The listing builds one solid part. Answer for the finished solid, in the listing's coordinates (mm). Face numbers are marked on the shaded views. Give positions to 0.01 mm unless a question says otherwise; leave off trailing zeros. Order: outer loops, then holes, each group sorted by start corner. A loop starts at its lowest first (then second) coordinate and runs counter-clockwise, first axis right, second up. Notation, with made-up numbers: (7.25, 17.5) - (16.25, 17.5) arc R27 ccw to (16.25, 33.5) - close; hole circle Ø8 at (7.25, 85). An arc over 180 degrees is marked (long way). Answer as a JSON object with one key per item and string values. Group by question number.
Q1. Consider line 1 (Y direction, x = 0, z = 2.7); line 2 (Z direction, x = 11, y = 2.25); line 3 (Z direction, x = 0, y = 2.5). Determine where each line is inside the solid, lowest interval first.
Q2. A cutting plane is placed at B-B, the plane z = 4. Give the vertices of the cut face in (x, y).
Q3. The mould has two halves that part along Y. Classify the marked faces 1, 2 and 3: released by +Y, released by -Y, zero draft, split by the parting line, or undercut.
Q4. A cutting plane is placed at A-A, the plane x = 13.5. Give the vertices of the cut face in (y, z).
Q5. Given pin 1 (0.8 mm diameter, centred on y = 3.5, z = 8, fed in from +X); pin 2 (3 mm diameter, centred on x = -14, y = 0, fed in from -Z); pin 3 (5 mm diameter, centred on x = -13, y = 2, fed in from +Z); pin 4 (5 mm diameter, centred on y = 3, z = 6.5, fed in from +X), each flat-ended and moving along its own axis, determine where each tip first touches the part or whether it passes through.
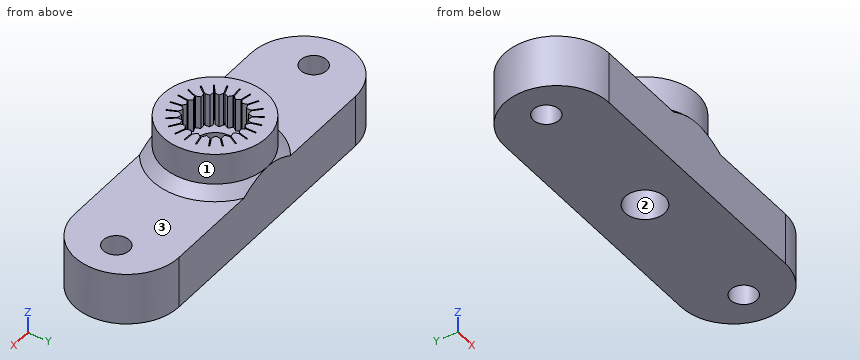
from build123d import *

# Parameters (mm, degrees)
EXTRUDE_1_DEPTH          = 5
SKETCH_6_R               = 5
EXTRUDE_3_DEPTH          = 4
CUT_EXTRUDE_5_DEPTH      = 3.2
CHAMFER_1_SIZE           = 1
CUT_EXTRUDE_6_DEPTH      = 21.303940504
CUT_EXTRUDE_6_DEPTH_BACK = 21.303940504
SKETCH_7_R               = 1.25
SKETCH_7_R_2             = 1.9


with BuildPart() as part:
    # ｽｹｯﾁ1 → ﾎﾞｽ - 押し出し1 (new body)
    with BuildSketch(Plane.XY):
        with BuildLine():
            Line((12.5, -5), (-12.5, -5))
            ThreePointArc((-12.5, -5), (-17.5, 0), (-12.5, 5))
            Line((-12.5, 5), (12.5, 5))
            ThreePointArc((12.5, 5), (17.5, 0), (12.5, -5))
        make_face()
    extrude(amount=EXTRUDE_1_DEPTH)

    # ｽｹｯﾁ6 → ﾎﾞｽ - 押し出し3 (add)
    with BuildSketch(Plane.XY.offset(5)):
        with Locations(Location((0, 0, 0), (0, 0, 270))):
            Circle(SKETCH_6_R)
    extrude(amount=EXTRUDE_3_DEPTH)

    # ｽｹｯﾁ5 → ｶｯﾄ - 押し出し5 (cut)
    with BuildSketch(Plane.XY.offset(9)):
        Polygon((-0.05, 2.95), (-0.05, 3.95), (0.05, 3.95), (0.05, 2.95), (0.362514094, 2.637485906), (0.747754611, 2.854095836), (1.017551382, 3.817013124), (1.11384311, 3.790033446), (0.844046339, 2.827116159), (1.060656269, 2.441875642), (1.490051682, 2.546516441), (2.009635632, 3.400935845), (2.095077573, 3.34897745), (1.575493623, 2.494558046), (1.680134421, 2.065162633), (2.121838437, 2.050073571), (2.852674402, 2.732626714), (2.920929716, 2.659543117), (2.190093752, 1.976989974), (2.17500469, 1.535285958), (2.596258142, 1.401586122), (3.484143361, 1.86165116), (3.530149865, 1.772862638), (2.642264646, 1.3127976), (2.50856481, 0.891544148), (2.878125258, 0.649149443), (3.857209346, 0.852605456), (3.877554947, 0.754697047), (2.898470859, 0.551241034), (2.656076155, 0.181680586), (2.94653499, -0.151431681), (3.944203759, -0.219674094), (3.937379518, -0.319440971), (2.939710748, -0.251198558), (2.606598481, -0.541657393), (2.796413701, -0.94078181), (3.738674623, -1.275661422), (3.705186662, -1.369887514), (2.76292574, -1.035007902), (2.363801323, -1.224823122), (2.4388952, -1.660358456), (3.255865093, -2.237038778), (3.198197061, -2.318735767), (2.381227168, -1.742055445), (1.945691834, -1.817149322), (1.900495, -2.25679391), (2.531582945, -3.032505201), (2.454011816, -3.095613995), (1.822923871, -2.319902705), (1.383279283, -2.274705871), (1.22114378, -2.685853285), (1.61954487, -3.603064586), (1.52782374, -3.642904695), (1.12942265, -2.725693394), (0.718275236, -2.563557891), (0.451225912, -2.915715208), (0.587392561, -3.906401154), (0.488323967, -3.920017819), (0.352157318, -2.929331873), (0, -2.66228255), (-0.352157318, -2.929331873), (-0.488323967, -3.920017819), (-0.587392561, -3.906401154), (-0.451225912, -2.915715208), (-0.718275236, -2.563557891), (-1.12942265, -2.725693394), (-1.52782374, -3.642904695), (-1.61954487, -3.603064586), (-1.22114378, -2.685853285), (-1.383279283, -2.274705871), (-1.822923871, -2.319902705), (-2.454011816, -3.095613995), (-2.531582945, -3.032505201), (-1.900495, -2.25679391), (-1.945691834, -1.817149322), (-2.381227168, -1.742055445), (-3.198197061, -2.318735767), (-3.255865093, -2.237038778), (-2.4388952, -1.660358456), (-2.363801323, -1.224823122), (-2.76292574, -1.035007902), (-3.705186662, -1.369887514), (-3.738674623, -1.275661422), (-2.796413701, -0.94078181), (-2.606598481, -0.541657393), (-2.939710748, -0.251198558), (-3.937379518, -0.319440971), (-3.944203759, -0.219674094), (-2.94653499, -0.151431681), (-2.656076155, 0.181680586), (-2.898470859, 0.551241034), (-3.877554947, 0.754697047), (-3.857209346, 0.852605456), (-2.878125258, 0.649149443), (-2.50856481, 0.891544148), (-2.642264646, 1.3127976), (-3.530149865, 1.772862638), (-3.484143361, 1.86165116), (-2.596258142, 1.401586122), (-2.17500469, 1.535285958), (-2.190093752, 1.976989974), (-2.920929716, 2.659543117), (-2.852674402, 2.732626714), (-2.121838437, 2.050073571), (-1.680134421, 2.065162633), (-1.575493623, 2.494558046), (-2.095077573, 3.34897745), (-2.009635632, 3.400935845), (-1.490051682, 2.546516441), (-1.060656269, 2.441875642), (-0.844046339, 2.827116159), (-1.11384311, 3.790033446), (-1.017551382, 3.817013124), (-0.747754611, 2.854095836), (-0.362514094, 2.637485906), align=None)
    extrude(amount=-CUT_EXTRUDE_5_DEPTH, mode=Mode.SUBTRACT)

    # 面取り1
    # the kernel refuses this chamfer: 1 mm, written as the material it adds along each edge
    with BuildSketch(Plane(origin=(0, 0, 5), x_dir=(0, -1, 0), z_dir=(-1, 0, 0))) as chamfer_1_piece_1_section:
        Polygon((5 + CHAMFER_1_SIZE, 0), (5, CHAMFER_1_SIZE), (5, 0), align=None)
    chamfer_1_piece_1 = revolve(axis=Axis((0, 0, 5), (0, 0, 1)), revolution_arc=180, mode=Mode.PRIVATE)
    chamfer_1_piece_1 = split(chamfer_1_piece_1, bisect_by=Plane(origin=(5.48673026, -5, 5.48673026), z_dir=(0, 1, 0)), keep=Keep.TOP, mode=Mode.PRIVATE)
    chamfer_1_piece_1 = split(chamfer_1_piece_1, bisect_by=Plane(origin=(5.48673026, 5, 5.48673026), z_dir=(0, -1, 0)), keep=Keep.TOP, mode=Mode.PRIVATE)
    add(chamfer_1_piece_1)
    with BuildSketch(Plane(origin=(0, 0, 5), x_dir=(0, 1, 0), z_dir=(1, 0, 0))) as chamfer_1_piece_2_section:
        Polygon((5 + CHAMFER_1_SIZE, 0), (5, CHAMFER_1_SIZE), (5, 0), align=None)
    chamfer_1_piece_2 = revolve(axis=Axis((0, 0, 5), (0, 0, 1)), revolution_arc=180, mode=Mode.PRIVATE)
    chamfer_1_piece_2 = split(chamfer_1_piece_2, bisect_by=Plane(origin=(-5.48673026, -5, 5.48673026), z_dir=(0, 1, 0)), keep=Keep.TOP, mode=Mode.PRIVATE)
    chamfer_1_piece_2 = split(chamfer_1_piece_2, bisect_by=Plane(origin=(-5.48673026, 5, 5.48673026), z_dir=(0, -1, 0)), keep=Keep.TOP, mode=Mode.PRIVATE)
    add(chamfer_1_piece_2)

    # ｽｹｯﾁ7 → ｶｯﾄ - 押し出し6 (cut, two sides: drawn at the far end of the back side and taken through both)
    with BuildSketch(Plane(origin=(0, 0, 0), x_dir=(-1, 0, 0), z_dir=(0, 0, -1)).offset(-CUT_EXTRUDE_6_DEPTH_BACK)):
        with Locations(Location((14, 0, 0), (0, 0, 180))):
            Circle(SKETCH_7_R)
        Circle(SKETCH_7_R_2)
        with Locations(Location((-14, 0, 0), (0, 0, 180))):
            Circle(SKETCH_7_R)
    extrude(amount=CUT_EXTRUDE_6_DEPTH + CUT_EXTRUDE_6_DEPTH_BACK, mode=Mode.SUBTRACT)


solid = part.part
Reply:
{
 "1": {"line 1": "y = -5 to -1.9, 1.9 to 5", "line 2": "z = 0 to 5", "line 3": "z = 0 to 5.8"},
 "2": {"outline": "(-12.5, -5) - (12.5, -5) arc R5 ccw to (12.5, 5) - (-12.5, 5) arc R5 ccw to start; hole circle Ø2.5 at (-14, 0); hole circle Ø3.8 at (0, 0); hole circle Ø2.5 at (14, 0)"},
 "3": {"face 1": "split by the parting line", "face 2": "undercut", "face 3": "zero draft"},
 "4": {"outline": "(-4.9, 0) - (-1.15, 0) - (-1.15, 5) - (-4.9, 5) - close; (1.15, 0) - (4.9, 0) - (4.9, 5) - (1.15, 5) - close"},
 "5": {"pin 1": "stops at x = 3.92", "pin 2": "stops at z = 0", "pin 3": "stops at z = 5", "pin 4": "stops at x = 17.4"}
}
